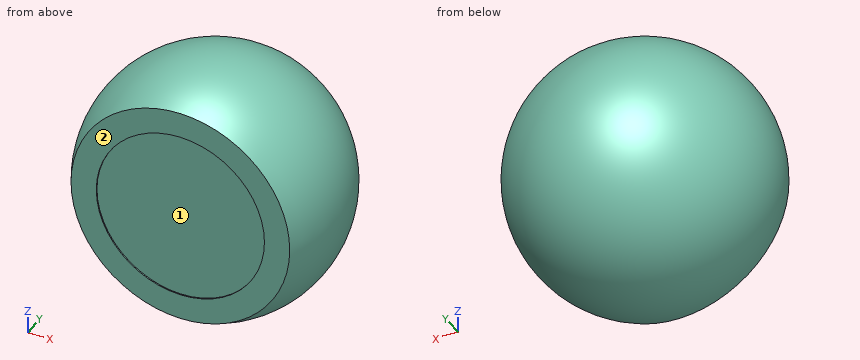
```python
from build123d import *

# Parameters (mm, degrees)
TRUNCATED_BALL_DEPTH      = 13.7
TRUNCATED_BALL_DEPTH_BACK = 13.7
SKETCH3_R                 = 8.4582
RECESSED_DEPTH            = 0.127


with BuildPart() as part:
    # Sketch1 → Complete_Ball (revolve)
    with BuildSketch(Plane.XY):
        with BuildLine():
            Line((0, 12.7), (0, -12.7))
            ThreePointArc((0, -12.7), (12.7, 0), (0, 12.7))
        make_face()
    revolve(axis=Axis((0, 13.6525, 0), (0, -1, 0)))

    # Sketch2 → Truncated_ball (cut, two sides)
    with BuildSketch(Plane.XY) as truncated_ball_sk:
        with BuildLine():
            Line((-10.998522628, -6.35), (10.998522628, -6.35))
            ThreePointArc((10.998522628, -6.35), (0, -12.7), (-10.998522628, -6.35))
        make_face()
    extrude(amount=TRUNCATED_BALL_DEPTH, mode=Mode.SUBTRACT)
    extrude(truncated_ball_sk.sketch, amount=-TRUNCATED_BALL_DEPTH_BACK, mode=Mode.SUBTRACT)

    # Sketch3 → Recessed (cut)
    with BuildSketch(Plane.XZ.offset(6.35)):
        with Locations(Location((0, 0, 0), (0, 0, 270))):  # turned: the seam where the file's is
            Circle(SKETCH3_R)
    extrude(amount=-RECESSED_DEPTH, mode=Mode.SUBTRACT)


solid = part.part
```
Model file for the job. Use its own axes, mm. Face numbers are marked on the shaded views. Coordinates: 2 decimals unless noted, no trailing zeros. Write each loop counter-clockwise with the first axis right and the second up, starting at its lowest first coordinate (ties: lowest second). Pieces come first, ordered by that corner, then holes. Notation, with made-up numbers: (12.5, -21) - (17.5, -21) arc R11 cw to (17.5, -2) - close; hole circle Ø7 at (41.5, 45.25). An arc over 180 degrees is marked (long way). Use a Markdown table: item, result. Add a question column.
Item 1: Band-saw the part on C-C, the plane y = 0.75. Write the cut outline in (x, z), and give its area (3 significant figures).
Item 2: Band-saw the part on D-D, the plane z = 10.5. Write the cut outline in (x, y).
Item 3: Drill centre lines: line 1 along X through (y, z) = (-6.3, 0); line 2 along X through (y, z) = (-2.75, 7); line 3 along Y through (x, z) = (6.25, -3.75). Where is each one in solid material? Low to high.
Item 4: Band-saw the part on A-A, the plane x = 0. Write the cut outline in (y, z).
Item 5: Drop flat-ended pins along their axis: pin 1 (5 mm diameter, centred on y = 8, z = -5.5, fed in from -X); pin 2 (1 mm diameter, centred on y = -1, z = 4.5, fed in from -X); pin 3 (4 mm diameter, centred on y = 1, z = -6.5, fed in from -X). Give the stop position or say it passes through.
Item 6: Band-saw the part on B-B, the plane z = 0. Write the cut outline in (x, y).
Item 7: Two-plate mould, pull along Z, no slides. Class the marked faces 1 and 2: pulls with the +Z half, pulls with the -Z half, needs draft (parallel to the pull), parting line crosses it, or undercut.
A:
| question | item | result |
|---|---|---|
| 1 | outline | circle Ø25.36 at (0, 0) |
| 1 | area | 505 mm² |
| 2 | outline | (-3.27, -6.35) - (3.27, -6.35) arc R7.14 ccw (long way) to start |
| 3 | line 1 | x = -11.03 to -8.46, 8.46 to 11.03 |
| 3 | line 2 | x = -10.23 to 10.23 |
| 3 | line 3 | y = -6.22 to 10.4 |
| 4 | outline | (-6.35, -11) arc R12.7 ccw (long way) to (-6.35, 11) - (-6.35, 8.46) - (-6.22, 8.46) - (-6.22, -8.46) - (-6.35, -8.46) - close |
| 5 | pin 1 | stops at x = -10.46 |
| 5 | pin 2 | stops at x = -12.02 |
| 5 | pin 3 | stops at x = -11.85 |
| 6 | outline | (-11, -6.35) - (-8.46, -6.35) - (-8.46, -6.22) - (8.46, -6.22) - (8.46, -6.35) - (11, -6.35) arc R12.7 ccw (long way) to start |
| 7 | face 1 | undercut |
| 7 | face 2 | needs draft |
